Model file for the job. Use its own axes, mm. A direction names the side the tool comes from. Round coordinates to 2 decimals unless told otherwise and drop trailing zeros. Loops run counter-clockwise (first coordinate to the right, second up) from the corner with the lowest first, then second, coordinate; pieces in that order, holes last. Notation, with made-up numbers: (83.5, 74) -> (122.5, 74) arc R18 cw to (122.5, 81) -> close; hole circle Ø5 at (26.5, 31.5). An arc over 180 degrees is marked (long way). Use a Markdown table: item, result.
from build123d import *

# Parameters (mm, degrees)
SKETCH1_R                               = 20
BOSS_EXTRUDE1_DEPTH                     = 50
SKETCH2_R                               = 40
BOSS_EXTRUDE2_DEPTH                     = 5
BOSS_EXTRUDE2_DRAFT                     = -1
CHAMFER1_SIZE                           = 2
CHAMFER1_SIZE2                          = 1.965988204
SKETCH3_R                               = 2.5
CUT_EXTRUDE1_DEPTH                      = 115.866956374
CIRPATTERN1_COUNT                       = 6
FILLET1_R                               = 3
CBORE_FOR_M5_HEX_HEAD_BOLT1_D           = 5.8
CBORE_FOR_M5_HEX_HEAD_BOLT1_CBORE_D     = 11
CBORE_FOR_M5_HEX_HEAD_BOLT1_CBORE_DEPTH = 0.5
MIRROR1_START                           = -50
MIRROR1_OUTLINE_R                       = 5.5
MIRROR1_DEPTH                           = 0.5
MIRROR1_3_OUTLINE_R                     = 2.5
MIRROR1_3_DEPTH                         = 5


with BuildPart() as part:
    # Sketch1 → Boss-Extrude1 (new, symmetric)
    with BuildSketch(Plane.XY):
        Circle(SKETCH1_R)
    extrude(amount=BOSS_EXTRUDE1_DEPTH, both=True)


with BuildPart() as boss_extrude2_tool:
    # Sketch2 → Boss-Extrude2 (with draft: the straight prism first)
    with BuildSketch(Plane.XY.offset(50)):
        Circle(SKETCH2_R)
    extrude(amount=-BOSS_EXTRUDE2_DEPTH)
    # Boss-Extrude2: the draft: its side faces are tilted about the plane it starts from
    boss_extrude2_sides = [boss_extrude2_tool.faces().sort_by_distance(p)[0] for p in [
        (-40, 0, 47.5),
    ]]
    draft(boss_extrude2_sides, Plane.XY.offset(50), BOSS_EXTRUDE2_DRAFT)


with BuildPart() as part_1:
    add(part.part)

    # Boss-Extrude2: add boss_extrude2_tool
    add(boss_extrude2_tool.part)

    # Chamfer1
    chamfer1_edges = [part_1.edges().sort_by_distance(p)[0] for p in [
        (-40, 0, 50),
    ]]
    chamfer1_side = [part_1.faces().sort_by_distance(p)[0] for p in [
        (-39.956362338, 0, 47.5),
    ]]
    chamfer(chamfer1_edges, length=CHAMFER1_SIZE, length2=CHAMFER1_SIZE2, reference=chamfer1_side[0])

    # Sketch3 → Cut-Extrude1 (cut, through all)
    with BuildSketch(Plane.XY.offset(50)):
        with Locations((0, 29.982547594)):
            Circle(SKETCH3_R)
    cut_extrude1 = extrude(amount=-CUT_EXTRUDE1_DEPTH, mode=Mode.SUBTRACT)

    # CirPattern1: Cut-Extrude1 ×6 about axis
    cirpattern1_axis = Axis((0, 0, 0), (0, 0, 1))
    for i in range(1, CIRPATTERN1_COUNT):
        add(cut_extrude1.rotate(cirpattern1_axis, i * 360 / CIRPATTERN1_COUNT), mode=Mode.SUBTRACT)

    # Fillet1
    fillet1_edges = [part_1.edges().sort_by_distance(p)[0] for p in [
        (-20, 0, 45),
    ]]
    fillet(fillet1_edges, radius=FILLET1_R)

    # CBORE for M5 Hex Head Bolt1 (through all)
    with Locations(Plane.XY.offset(50)):
        with Locations((0, 0)):
            CounterBoreHole(CBORE_FOR_M5_HEX_HEAD_BOLT1_D / 2, CBORE_FOR_M5_HEX_HEAD_BOLT1_CBORE_D / 2, CBORE_FOR_M5_HEX_HEAD_BOLT1_CBORE_DEPTH)

    # Mirror1: read off the stored shape, not the designer's step
    # Mirror1 outline → Mirror1 (cut)
    with BuildSketch(Plane.XY.offset(MIRROR1_START)):
        Circle(MIRROR1_OUTLINE_R)
    extrude(amount=MIRROR1_DEPTH, mode=Mode.SUBTRACT)

    # Mirror1 2 outline → Mirror1 2 (revolve)
    with BuildSketch(Plane.XZ):
        with BuildLine():
            Line((38, -50), (39.965688775, -48.034311225))
            Line((39.965688775, -48.034311225), (39.912724675, -45))
            Line((39.912724675, -45), (23, -45))
            ThreePointArc((23, -45), (20.878679656, -44.121320344), (20, -42))
            Line((20, -42), (20, -50))
            Line((20, -50), (38, -50))
        make_face()
    revolve(axis=Axis((0, 0, 0), (0, 0, 1)))

    # Mirror1 3 outline → Mirror1 3 (cut)
    with BuildSketch(Plane.XY.offset(MIRROR1_START)):
        with Locations((0, 29.982547594)):
            Circle(MIRROR1_3_OUTLINE_R)
        with Locations((25.965647886, 14.991273797)):
            Circle(MIRROR1_3_OUTLINE_R)
        with Locations((25.965647886, -14.991273797)):
            Circle(MIRROR1_3_OUTLINE_R)
        with Locations((0, -29.982547594)):
            Circle(MIRROR1_3_OUTLINE_R)
        with Locations((-25.965647886, -14.991273797)):
            Circle(MIRROR1_3_OUTLINE_R)
        with Locations((-25.965647886, 14.991273797)):
            Circle(MIRROR1_3_OUTLINE_R)
    extrude(amount=MIRROR1_3_DEPTH, mode=Mode.SUBTRACT)


solid = part_1.part
Q1. Pull direction X, two halves, no side cores. Call faces 1 (the face through (-8.655, -38.978, -45.822)), 2 (the face through (-1.19, -5.37, -49.75)), 3 (the face through (17, -17, 45)): released by +X, released by -X, zero draft, split by the parting line, or undercut.
Results list:
| item | result |
|---|---|
| face 1 | split by the parting line |
| face 2 | undercut |
| face 3 | zero draft |
Q2. Band-saw the part on A-A, the plane z = -21. Give the cut face in (x, y), plus the area to 3 significant figures.
Results list:
| item | result |
|---|---|
| outline | circle Ø40 at (0, 0); hole circle Ø5.8 at (0, 0) |
| area | 1,230 mm² |
Q3. Tool access for faces 4 (the face through (1.154, 27.765, 47.535)), 5 (the face through (17, -17, -45)): list every direction of +Z, -Z, +X, -X, +Y, -Y with a clear straight run to the whole face (end or side of a thin tool).
Results list:
| item | result |
|---|---|
| face 4 | +Z, -Z |
| face 5 | none |
Q4. Flat gauge pins, fed straight in: pin 1 (1.5 mm diameter, centred on x = -11.5, z = -14.5, fed in from -Y); pin 2 (6.5 mm diameter, centred on x = 0, y = 0, fed in from +Z); pin 3 (6 mm diameter, centred on y = 11, z = 32.5, fed in from +X); pin 4 (4.5 mm diameter, centred on x = 0, y = 0, fed in from -Z). Where does each tip first touch, or does it go through?
Results list:
| item | result |
|---|---|
| pin 1 | stops at y = -16.87 |
| pin 2 | stops at z = 49.5 |
| pin 3 | stops at x = 18.33 |
| pin 4 | passes through |
Q5. Band-saw the part on B-B, the plane x = 0. Give the number of separate pieces and of enclosed holes in the cut face, plus the area to 3 significant figures.
Results list:
| item | result |
|---|---|
| separate pieces | 6 |
| enclosed holes | 0 |
| area | 3,710 mm² |
Q6. Drill centre lines: L1, parallel to Y at x = 0, z = -19; L2, parallel to Y at x = 0, z = -49.75; L3, parallel to Z at x = -14.5, y = -26. Where is each one in solid material? Low to high. Write a range as from..to.
Results list:
| item | result |
|---|---|
| L1 | y = -20..-2.9, 2.9..20 |
| L2 | y = -38.25..-32.48, -27.48..-5.5, 5.5..27.48, 32.48..38.25 |
| L3 | z = -50..-45, 45..50 |
